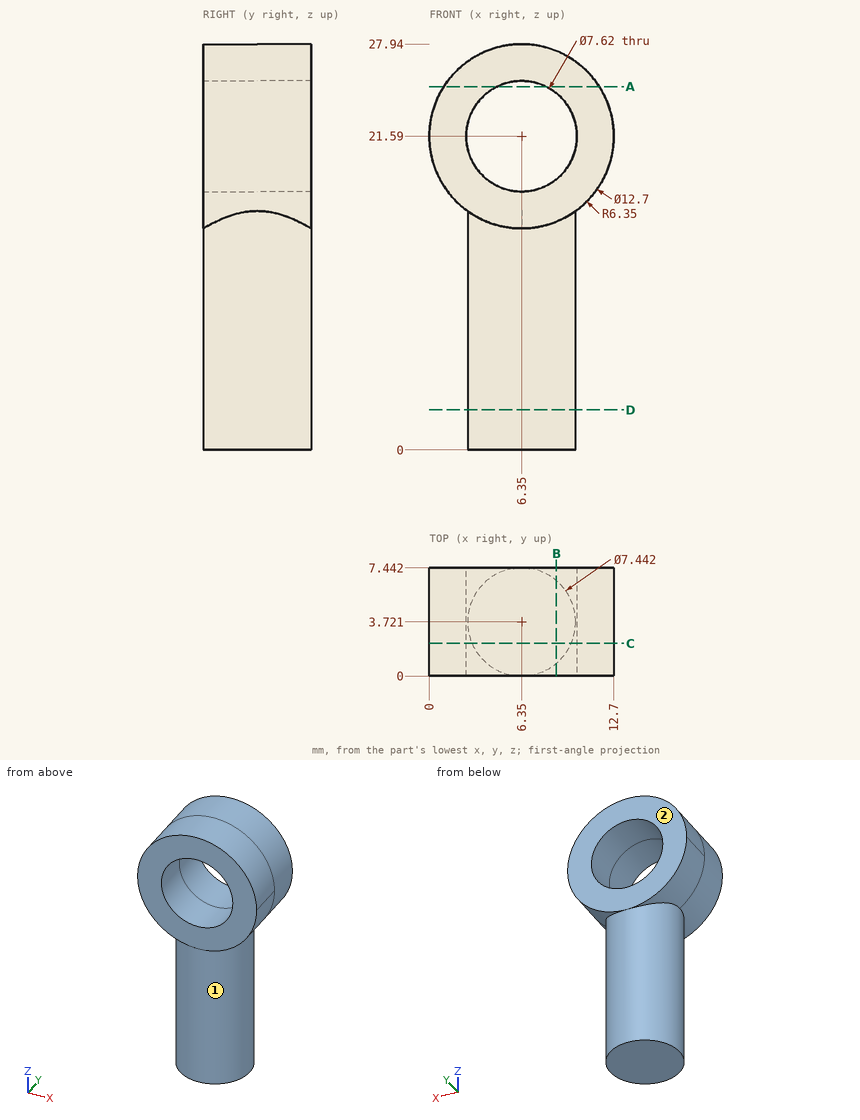
Answer from the drawing. Dimensions are ordinates in mm from the lowest x, y and z of the part. A direction names the side the tool comes from. Coordinates: 2 decimals unless noted, no trailing zeros. Write each loop counter-clockwise with the first axis right and the second up, starting at its lowest first coordinate (ties: lowest second). Pieces come first, ordered by that corner, then holes. Notation, with made-up numbers: M 33,46.25 L 55,46.25 A32 cw 55,80.25 Z; hole C 8.5,-36 d7. An arc over 180 degrees is marked long. Use one line per item in the form item = value. Start each with the question number.
1. Each of these flat-tipped pins is pushed along its axis until it touches: P1, Ø4, axis at y = 5, z = 4.5, coming from the -X side; P2, Ø4, axis at x = 2.5, z = 5, coming from the +Y side; P3, Ø5, axis at x = 10, z = 12.5, coming from the +Y side. Where does it stop, or does it pass through?
2. A tool of negligible diameter and unlimited length cuts with its end or side. For the marked faces 1 and 2, from which of +Z, -Z, +X, -X, +Y, -Y can it reach the whole face along a straight path? Write none if from no direction.
3. Straight lines are drawn through the part: probe 1 along X at (y, z) = (1.5, 21.75); probe 2 along Z at (x, y) = (6.35, 6.45); probe 3 along Z at (x, y) = (3, 3.75) (1 decimal). For each, find the intervals that lie inside material, in ascending order. Write a range as from..to.
4. The part is cut by section C-C (y = 2.25). Give the vertices of the cut face in (x, z), plus the area to 3 significant figures.
5. The part is cut by section B-B (x = 8.75). Give the vertices of the cut face in (y, z) (1 decimal).
6. The part is cut by section D-D (z = 2.75). Give the vertices of the cut face in (x, y).
7. The part is cut by section A-A (z = 25). Give the vertices of the cut face in (x, y).
Evaluation:
q1.P1 = 2.63
q1.P2 = 6.95
q1.P3 = 7.26
q2.face_1 = -Z
q2.face_2 = +Z, -Z, +X, -X, +Y
q3.probe_1 = 0..2.54, 10.16..12.7
q3.probe_2 = 0..17.78, 25.4..27.94
q3.probe_3 = 0..19.8, 23.4..27
q4.outline = M 2.93,0 L 9.77,0 L 9.77,16.24 A6.35 ccw long 2.93,16.24 Z; hole C 6.35,21.59 d7.62
q4.area = 187 mm^2
q5.outline = M 0,15.7 L 0.9,15.7 L 0.9,0 L 6.6,0 L 6.6,15.7 L 7.4,15.7 L 7.4,18.6 L 0,18.6 Z; M 0,24.5 L 7.4,24.5 L 7.4,27.5 L 0,27.5 Z
q6.outline = C 6.35,3.72 d7.44
q7.outline = M 0.99,0 L 4.65,0 L 4.65,7.44 L 0.99,7.44 Z; M 8.05,0 L 11.71,0 L 11.71,7.44 L 8.05,7.44 Z
